Here's how the part is built. I have some questions about the finished solid (model axes, mm). A direction names the side the tool comes from. Round coordinates to 2 decimals unless told otherwise and drop trailing zeros. Order: outer loops, then holes, each group sorted by start corner. A loop starts at its lowest first (then second) coordinate and runs counter-clockwise, first axis right, second up. Notation, with made-up numbers: (21.25, 78) -> (41.25, 78) arc R23 cw to (41.25, 103) -> close; hole circle Ø3 at (-2, 28). An arc over 180 degrees is marked (long way). Answer in a Markdown table with one row per item.
```python
from build123d import *

# Parameters (mm, degrees)
BOSS_EXTRUDE1_DEPTH = 14
BOSS_EXTRUDE2_DEPTH = 18
CUT_EXTRUDE1_START  = -15
CUT_EXTRUDE1_DEPTH  = 15
FILLET4_R           = 1
FILLET5_R           = 0.5


with BuildPart() as part:
    # Sketch1 → Boss-Extrude1 (new body)
    with BuildSketch(Plane(origin=(0, 0, 0), x_dir=(1, 0, 0), z_dir=(0, 1, 0))):
        with BuildLine():
            Line((-2.1, 3.1), (2.1, 3.1))
            ThreePointArc((2.1, 3.1), (2.807106781, 2.807106781), (3.1, 2.1))
            Line((3.1, 2.1), (3.1, -2.1))
            ThreePointArc((3.1, -2.1), (2.807106781, -2.807106781), (2.1, -3.1))
            Line((2.1, -3.1), (-2.1, -3.1))
            ThreePointArc((-2.1, -3.1), (-2.807106781, -2.807106781), (-3.1, -2.1))
            Line((-3.1, -2.1), (-3.1, 2.1))
            ThreePointArc((-3.1, 2.1), (-2.807106781, 2.807106781), (-2.1, 3.1))
        make_face()
    extrude(amount=BOSS_EXTRUDE1_DEPTH)

    # Sketch2 → Boss-Extrude2 (add)
    with BuildSketch(Plane(origin=(0, 14, 0), x_dir=(1, 0, 0), z_dir=(0, 1, 0))):
        with BuildLine():
            Line((-2.2, 5.2), (2.2, 5.2))
            ThreePointArc((2.2, 5.2), (4.321320344, 4.321320344), (5.2, 2.2))
            Line((5.2, 2.2), (5.2, -2.2))
            ThreePointArc((5.2, -2.2), (4.321320344, -4.321320344), (2.2, -5.2))
            Line((2.2, -5.2), (-2.2, -5.2))
            ThreePointArc((-2.2, -5.2), (-4.321320344, -4.321320344), (-5.2, -2.2))
            Line((-5.2, -2.2), (-5.2, 2.2))
            ThreePointArc((-5.2, 2.2), (-4.321320344, 4.321320344), (-2.2, 5.2))
        make_face()
    extrude(amount=BOSS_EXTRUDE2_DEPTH)

    # Sketch3 → Cut-Extrude1 (cut)
    with BuildSketch(Plane(origin=(0, 32, 0), x_dir=(1, 0, 0), z_dir=(0, 1, 0)).offset(CUT_EXTRUDE1_START)):
        with BuildLine():
            Line((-2.1, 3.1), (2.1, 3.1))
            ThreePointArc((2.1, 3.1), (2.807106781, 2.807106781), (3.1, 2.1))
            Line((3.1, 2.1), (3.1, -2.1))
            ThreePointArc((3.1, -2.1), (2.807106781, -2.807106781), (2.1, -3.1))
            Line((2.1, -3.1), (-2.1, -3.1))
            ThreePointArc((-2.1, -3.1), (-2.807106781, -2.807106781), (-3.1, -2.1))
            Line((-3.1, -2.1), (-3.1, 2.1))
            ThreePointArc((-3.1, 2.1), (-2.807106781, 2.807106781), (-2.1, 3.1))
        make_face()
    extrude(amount=CUT_EXTRUDE1_DEPTH, mode=Mode.SUBTRACT)

    # Fillet4
    fillet4_edges = [part.edges().sort_by_distance(p)[0] for p in [
        (-4.321320344, 14, 4.321320344),
        (0, 14, 5.2),
        (4.321320344, 14, 4.321320344),
        (5.2, 14, 0),
        (4.321320344, 14, -4.321320344),
        (0, 14, -5.2),
        (-4.321320344, 14, -4.321320344),
        (-5.2, 14, 0),
    ]]
    fillet(fillet4_edges, radius=FILLET4_R)

    # Fillet5
    fillet5_edges = [part.edges().sort_by_distance(p)[0] for p in [
        (0, 0, -3.1),
        (2.807106781, 0, -2.807106781),
        (3.1, 0, 0),
        (2.807106781, 0, 2.807106781),
        (0, 0, 3.1),
        (-2.807106781, 0, 2.807106781),
        (-3.1, 0, 0),
        (-2.807106781, 0, -2.807106781),
    ]]
    fillet(fillet5_edges, radius=FILLET5_R)


solid = part.part
```
1. Suppose I cut it at D-D on y = 15.5. Write out the boundary of the cut face in (x, z).
Numbers:
| item | result |
|---|---|
| outline | (-5.2, -2.2) arc R3 ccw to (-2.2, -5.2) -> (2.2, -5.2) arc R3 ccw to (5.2, -2.2) -> (5.2, 2.2) arc R3 ccw to (2.2, 5.2) -> (-2.2, 5.2) arc R3 ccw to (-5.2, 2.2) -> close |
2. Please list where these lines run through material, in increasing order: line 1 along X through (y, z) = (19, -0.75); line 2 along Z through (x, y) = (1.75, 10).
Numbers:
| item | result |
|---|---|
| line 1 | x = -5.2 to -3.1, 3.1 to 5.2 |
| line 2 | z = -3.1 to 3.1 |
3. Suppose I cut it at B-B on z = -1. Write out the boundary of the cut face in (x, y), then the cut area to 3 significant figures.
Numbers:
| item | result |
|---|---|
| outline | (-5.2, 15) arc R1 ccw to (-4.2, 14) -> (-3.1, 14) -> (-3.1, 0.5) arc R0.5 ccw to (-2.6, 0) -> (2.6, 0) arc R0.5 ccw to (3.1, 0.5) -> (3.1, 14) -> (4.2, 14) arc R1 ccw to (5.2, 15) -> (5.2, 32) -> (3.1, 32) -> (3.1, 17) -> (-3.1, 17) -> (-3.1, 32) -> (-5.2, 32) -> close |
| area | 180 mm2 |
4. We'd pull the mould along X, two halves only. Please class faces 4 (the face through (3.1, 24, 0)), 5 (the face through (0, 23, -5.2)), 6 (the face through (4.3, 23.38, -4.34)), 7 (the face through (0, 24, 3.1)): released by +X, released by -X, zero draft, split by the parting line, or undercut.
Numbers:
| item | result |
|---|---|
| face 4 | undercut |
| face 5 | zero draft |
| face 6 | released by +X |
| face 7 | undercut |
5. For pin 1 Ø3.5 at (y, z) = (4, 1) entering from -X; pin 2 Ø3 at (x, z) = (-1.5, 0.5) entering from +Y; pin 3 Ø1 at (x, y) = (-3, 8) entering from +Z, each with a flat end and sliding along its axis, tell me the tip position at first contact or that it passes through.
Numbers:
| item | result |
|---|---|
| pin 1 | stops at x = -3.1 |
| pin 2 | stops at y = 17 |
| pin 3 | stops at z = 3.02 |
6. Suppose I cut it at C-C on x = -1.25. Write out the boundary of the cut face in (y, z), then the cut area to 3 significant figures.
Numbers:
| item | result |
|---|---|
| outline | (0, -2.6) arc R0.5 ccw to (0.5, -3.1) -> (14, -3.1) -> (14, -4.2) arc R1 ccw to (15, -5.2) -> (32, -5.2) -> (32, -3.1) -> (17, -3.1) -> (17, 3.1) -> (32, 3.1) -> (32, 5.2) -> (15, 5.2) arc R1 ccw to (14, 4.2) -> (14, 3.1) -> (0.5, 3.1) arc R0.5 ccw to (0, 2.6) -> close |
| area | 180 mm2 |
7. Suppose I cut it at A-A on y = 24. Write out the boundary of the cut face in (x, z).
Numbers:
| item | result |
|---|---|
| outline | (-5.2, -2.2) arc R3 ccw to (-2.2, -5.2) -> (2.2, -5.2) arc R3 ccw to (5.2, -2.2) -> (5.2, 2.2) arc R3 ccw to (2.2, 5.2) -> (-2.2, 5.2) arc R3 ccw to (-5.2, 2.2) -> close; hole (-3.1, -2.1) arc R1 ccw to (-2.1, -3.1) -> (2.1, -3.1) arc R1 ccw to (3.1, -2.1) -> (3.1, 2.1) arc R1 ccw to (2.1, 3.1) -> (-2.1, 3.1) arc R1 ccw to (-3.1, 2.1) -> close |
8. For faces 1 (the face through (-2.815, 7.156, -2.799)), 2 (the face through (-2.799, 24.395, 2.815)), 3 (the face through (2.799, 7.156, -2.815)), which set-ups out of +Z, -Z, +X, -X, +Y, -Y let a thin tool reach every point of the face, with its end or its side?
Numbers:
| item | result |
|---|---|
| face 1 | -Z, -X, -Y |
| face 2 | +Y |
| face 3 | -Z, +X, -Y |
